CAD build for the part. Positions are in the model's coordinates, mm. A direction names the side the tool comes from. Give positions to 0.01 mm unless a question says otherwise; leave off trailing zeros. Write each loop counter-clockwise with the first axis right and the second up, starting at its lowest first coordinate (ties: lowest second). Pieces come first, ordered by that corner, then holes. Notation, with made-up numbers: (58, -19) -> (90, -19) arc R23 ccw to (90, 19) -> close; hole circle Ø6 at (30, -18). An arc over 180 degrees is marked (long way). Answer in a Markdown table with one row per item. Add a question column.
```python
from build123d import *

# Parameters (mm, degrees)
F1_DEPTH      = 152.4
F2_R          = 12.7
F3_W          = 6.35
F3_H          = 76.2
F4_DEPTH      = 38.101
F4_DEPTH_BACK = 38.101


with BuildPart() as f1:
    # F0 (on Front) → F1 (new body)
    with BuildSketch(Plane.XZ):
        with BuildLine():
            Line((-6.35, 93.9159601581), (-6.35, 81.2159601581))
            Line((-6.35, 81.2159601581), (-38.1, 81.2159601581))
            Line((-38.1, 81.2159601581), (-38.1, 5.0159601581))
            Line((-38.1, 5.0159601581), (-9.9460958472, 1.3094283595))
            ThreePointArc((-9.9460958472, 1.3094283595), (0, 0.6575267962), (9.9460958472, 1.3094283595))
            Line((9.9460958472, 1.3094283595), (38.1, 5.0159601581))
            Line((38.1, 5.0159601581), (38.1, 81.2159601581))
            Line((38.1, 81.2159601581), (6.35, 81.2159601581))
            Line((6.35, 81.2159601581), (6.35, 93.9159601581))
            Line((6.35, 93.9159601581), (-6.35, 93.9159601581))
        make_face()
    extrude(amount=F1_DEPTH)

    # F2
    f2_edges = [f1.edges().sort_by_distance(p)[0] for p in [
        (38.1, -76.2, 81.21596),
        (-38.1, -76.2, 81.21596),
        (-38.1, -76.2, 5.01596),
        (38.1, -76.2, 5.01596),
    ]]
    fillet(f2_edges, radius=F2_R)

    # F3 (on Right) → F4 (cut, two sides)
    with BuildSketch(Plane.YZ) as f4_sk:
        with Locations((-98.425, 33.0594283595)):
            Rectangle(F3_W, F3_H)
    extrude(amount=-F4_DEPTH, mode=Mode.SUBTRACT)
    extrude(f4_sk.sketch, amount=F4_DEPTH_BACK, mode=Mode.SUBTRACT)


solid = f1.part
```
Item 1: Probe L1, parallel to Y at x = -23, z = 12.5; L2, parallel to Z at x = 0.5, y = -20; L3, parallel to X at y = -81.5, z = 84.5. List the from-to ranges inside material, lowest first. Write a range as from..to.
Item 2: Slice it at A-A, the plane z = 34. List the corners of the cut face in (x, y).
Item 3: Which spindle directions (+Z, -Z, +X, -X, +Y, -Y) get a long thin tool onto all of the face, cutting with end or side? Do faces 4 (the face through (-6.35, -75, 88)), 5 (the face through (1, -95.25, 35)), 6 (the face through (16, -75, 81.216)). Say none if no direction does.
Item 4: Drop flat-ended pins along their axis: pin 1 Ø6.5 at (y, z) = (-39.5, 89) entering from -X; pin 2 Ø12 at (x, z) = (17.5, 15) entering from +Y; pin 3 Ø4 at (y, z) = (-94.5, 87.5) entering from +X; pin 4 Ø9.5 at (x, y) = (-18, -85) entering from +Z. Give the stop position or say it passes through.
Item 5: Mould opens along Y. For faces 1 (the face through (1, -101.6, 35)), 2 (the face through (-1, 0, 48)), 3 (the face through (-38.1, -127, 43)) say: released by +Y, released by -Y, zero draft, split by the parting line, or undercut.
Item 6: Slice it at B-B, the plane y = -62. List the corners of the cut face in (x, z).
Item 7: Slice it at C-C, the plane x = 30. List the corners of the cut face in (y, z), then the cut area to 3 significant figures.
Item 8: Slice it at D-D, the plane z = 12.5. List the corners of the cut face in (x, y).
Answer key:
| question | item | result |
|---|---|---|
| 1 | L1 | y = -152.4..-101.6, -95.25..0 |
| 1 | L2 | z = 0.66..93.92 |
| 1 | L3 | x = -6.35..6.35 |
| 2 | outline | (-38.1, -152.4) -> (38.1, -152.4) -> (38.1, -101.6) -> (-38.1, -101.6) -> close; (-38.1, -95.25) -> (38.1, -95.25) -> (38.1, 0) -> (-38.1, 0) -> close |
| 3 | face 4 | +Z, -X, +Y, -Y |
| 3 | face 5 | -Z, +X, -X |
| 3 | face 6 | +Z, +X, +Y, -Y |
| 4 | pin 1 | stops at x = -6.35 |
| 4 | pin 2 | stops at y = 0 |
| 4 | pin 3 | stops at x = 6.35 |
| 4 | pin 4 | stops at z = 81.22 |
| 5 | face 1 | undercut |
| 5 | face 2 | released by +Y |
| 5 | face 3 | zero draft |
| 6 | outline | (-38.1, 16.15) arc R12.7 ccw to (-27.06, 3.56) -> (-9.95, 1.31) arc R76.2 ccw to (9.95, 1.31) -> (27.06, 3.56) arc R12.7 ccw to (38.1, 16.15) -> (38.1, 68.52) arc R12.7 ccw to (25.4, 81.22) -> (6.35, 81.22) -> (6.35, 93.92) -> (-6.35, 93.92) -> (-6.35, 81.22) -> (-25.4, 81.22) arc R12.7 ccw to (-38.1, 68.52) -> close |
| 7 | outline | (-152.4, 4.32) -> (-101.6, 4.32) -> (-101.6, 71.16) -> (-95.25, 71.16) -> (-95.25, 4.32) -> (0, 4.32) -> (0, 80.35) -> (-152.4, 80.35) -> close |
| 7 | area | 11,200 mm² |
| 8 | outline | (-37.56, -152.4) -> (37.56, -152.4) -> (37.56, -101.6) -> (-37.56, -101.6) -> close; (-37.56, -95.25) -> (37.56, -95.25) -> (37.56, 0) -> (-37.56, 0) -> close |
